Check sheet for the modelled part. Datum: model origin and axes. Units: mm. A direction names the side the tool comes from. Round coordinates to 2 decimals unless told otherwise and drop trailing zeros. Loops run counter-clockwise (first coordinate to the right, second up) from the corner with the lowest first, then second, coordinate; pieces in that order, holes last. Notation, with made-up numbers: (-27.75, -3.5) -> (18.25, -3.5) arc R26 cw to (18.25, 24.5) -> close; hole circle Ø2 at (48, -16.5). An arc over 180 degrees is marked (long way). One line per item, written item: value. Start each with the question number.
1. Release check for a two-part mould opening along X. For faces 1 (the face through (2.01, 3.46, 0.99)), 2 (the face through (-4.8, 1.67, 0.99)), 3 (the face through (-1.99, 3.47, 0.99)), 4 (the face through (0, 6, 1)) record: +X half, -X half, draft (parallel to the pull), parting line (faces both ways), or undercut.
2. Cross-section at D-D on y = -3. Record the cut outline in (x, z), then the cut area to 3 significant figures.
3. Set-up check for faces 5 (the face through (-4.77, -1.64, 0.99)), 6 (the face through (3.84, 3.32, 0.99)), 7 (the face through (4.77, 1.64, 0.99)): record each of +Z, -Z, +X, -X, +Y, -Y from which the full face is reachable in a straight line by a thin tool's end or side.
4. Material ranges on L1, parallel to Y at x = 0, z = 0.8; L2, parallel to Y at x = -4.5, z = 1.9; L3, parallel to X at y = 5, z = 1.85, recorded low to high.
5. Cross-section at B-B on z = 1.4. Record the cut outline in (x, y).
6. Cross-section at A-A on x = 0. Record the cut outline in (y, z), then the cut area to 3 significant figures.
7. Cross-section at C-C on y = 0.5. Record the cut outline in (x, z).
8. Go/stop test with a flat-tipped pin: pin 1 (1.8 mm diameter, centred on x = 0, y = 0, fed in from -Z). Record where the tip stops, or that it passes through.
from build123d import *

# Parameters (mm, degrees)
F1_DEPTH = 2
F2_R     = 1
F3_DEPTH = 2.001


with BuildPart() as f1:
    # F0 (on Top) → F1 (new body)
    with BuildSketch(Plane.XY):
        with BuildLine():
            ThreePointArc((3.877013, -0.984261), (3.969134, -0.495958), (4, 0))
            ThreePointArc((4, 0), (3.969134, 0.495958), (3.877013, 0.984261))
            ThreePointArc((3.877013, 0.984261), (3.464102, 2), (2.790902, 2.865461))
            ThreePointArc((2.790902, 2.865461), (2, 3.464102), (1.086111, 3.849722))
            ThreePointArc((1.086111, 3.849722), (0.548229, 3.962252), (0, 4))
            ThreePointArc((0, 4), (-0.548229, 3.962252), (-1.086111, 3.849722))
            ThreePointArc((-1.086111, 3.849722), (-2, 3.464102), (-2.790902, 2.865461))
            ThreePointArc((-2.790902, 2.865461), (-3.464102, 2), (-3.877013, 0.984261))
            ThreePointArc((-3.877013, 0.984261), (-4, 0), (-3.877013, -0.984261))
            ThreePointArc((-3.877013, -0.984261), (-3.464102, -2), (-2.790902, -2.865461))
            ThreePointArc((-2.790902, -2.865461), (-2, -3.464102), (-1.086111, -3.849722))
            ThreePointArc((-1.086111, -3.849722), (0, -4), (1.086111, -3.849722))
            ThreePointArc((1.086111, -3.849722), (2, -3.464102), (2.790902, -2.865461))
            ThreePointArc((2.790902, -2.865461), (3.464102, -2), (3.877013, -0.984261))
        make_face()
        with BuildLine():
            ThreePointArc((2.790902, 2.865461), (3.464102, 2), (3.877013, 0.984261))
            ThreePointArc((3.877013, 0.984261), (4.783962, 1.654296), (5.446152, 2.566987))
            Line((5.446152, 2.566987), (5.196152, 3))
            Line((5.196152, 3), (4.946152, 3.433013))
            ThreePointArc((4.946152, 3.433013), (3.824643, 3.315885), (2.790902, 2.865461))
        make_face()
        with BuildLine():
            ThreePointArc((5.446152, -2.566987), (4.783962, -1.654296), (3.877013, -0.984261))
            ThreePointArc((3.877013, -0.984261), (3.464102, -2), (2.790902, -2.865461))
            ThreePointArc((2.790902, -2.865461), (3.824643, -3.315885), (4.946152, -3.433013))
            Line((4.946152, -3.433013), (5.196152, -3))
            Line((5.196152, -3), (5.446152, -2.566987))
        make_face()
        with BuildLine():
            ThreePointArc((0, 4), (0.548229, 3.962252), (1.086111, 3.849722))
            ThreePointArc((1.086111, 3.849722), (0.959319, 4.97018), (0.5, 6))
            Line((0.5, 6), (0, 6))
            Line((0, 6), (0, 4))
        make_face()
        with BuildLine():
            ThreePointArc((0.5, -6), (0.959319, -4.97018), (1.086111, -3.849722))
            ThreePointArc((1.086111, -3.849722), (0, -4), (-1.086111, -3.849722))
            ThreePointArc((-1.086111, -3.849722), (-0.959319, -4.97018), (-0.5, -6))
            Line((-0.5, -6), (0, -6))
            Line((0, -6), (0.5, -6))
        make_face()
        with BuildLine():
            ThreePointArc((-1.086111, 3.849722), (-0.548229, 3.962252), (0, 4))
            Line((0, 4), (0, 6))
            Line((0, 6), (-0.5, 6))
            ThreePointArc((-0.5, 6), (-0.959319, 4.97018), (-1.086111, 3.849722))
        make_face()
        with BuildLine():
            ThreePointArc((-4.946152, -3.433013), (-3.824643, -3.315885), (-2.790902, -2.865461))
            ThreePointArc((-2.790902, -2.865461), (-3.464102, -2), (-3.877013, -0.984261))
            ThreePointArc((-3.877013, -0.984261), (-4.783962, -1.654296), (-5.446152, -2.566987))
            Line((-5.446152, -2.566987), (-5.196152, -3))
            Line((-5.196152, -3), (-4.946152, -3.433013))
        make_face()
        with BuildLine():
            ThreePointArc((-3.877013, 0.984261), (-3.464102, 2), (-2.790902, 2.865461))
            ThreePointArc((-2.790902, 2.865461), (-3.824643, 3.315885), (-4.946152, 3.433013))
            Line((-4.946152, 3.433013), (-5.196152, 3))
            Line((-5.196152, 3), (-5.446152, 2.566987))
            ThreePointArc((-5.446152, 2.566987), (-4.783962, 1.654296), (-3.877013, 0.984261))
        make_face()
    extrude(amount=F1_DEPTH)

    # F2 (on face) → F3 (cut, through all)
    with BuildSketch(Plane.XY.offset(2)):
        Circle(F2_R)
    extrude(amount=-F3_DEPTH, mode=Mode.SUBTRACT)


solid = f1.part
Taken from the geometry:
1. face 1: undercut
1. face 2: -X half
1. face 3: undercut
1. face 4: draft
2. outline: (-5.2, 0) -> (-3.02, 0) -> (-3.02, 2) -> (-5.2, 2) -> close; (-2.65, 0) -> (2.65, 0) -> (2.65, 2) -> (-2.65, 2) -> close; (3.02, 0) -> (5.2, 0) -> (5.2, 2) -> (3.02, 2) -> close
2. area: 19.3 mm2
3. face 5: +Z, -Z, -X
3. face 6: +Z, -Z, +Y
3. face 7: +Z, -Z, +X
4. L1: y = -6 to -1, 1 to 6
4. L2: y = -3.43 to -1.4, 1.4 to 3.43
4. L3: x = -0.95 to 0.95
5. outline: (-5.45, -2.57) -> (-4.95, -3.43) arc R3.69 ccw to (-2.79, -2.87) arc R4 ccw to (-1.09, -3.85) arc R3.69 ccw to (-0.5, -6) -> (0.5, -6) arc R3.69 ccw to (1.09, -3.85) arc R4 ccw to (2.79, -2.87) arc R3.69 ccw to (4.95, -3.43) -> (5.45, -2.57) arc R3.69 ccw to (3.88, -0.98) arc R4 ccw to (4, 0) arc R4 ccw to (3.88, 0.98) arc R3.69 ccw to (5.45, 2.57) -> (4.95, 3.43) arc R3.69 ccw to (2.79, 2.87) arc R4 ccw to (1.09, 3.85) arc R3.69 ccw to (0.5, 6) -> (-0.5, 6) arc R3.69 ccw to (-1.09, 3.85) arc R4 ccw to (-2.79, 2.87) arc R3.69 ccw to (-4.95, 3.43) -> (-5.45, 2.57) arc R3.69 ccw to (-3.88, 0.98) arc R4 ccw to (-3.88, -0.98) arc R3.69 ccw to start; hole circle Ø2 at (0, 0)
6. outline: (-6, 0) -> (-1, 0) -> (-1, 2) -> (-6, 2) -> close; (1, 0) -> (6, 0) -> (6, 2) -> (1, 2) -> close
6. area: 20.0 mm2
7. outline: (-3.97, 0) -> (-0.87, 0) -> (-0.87, 2) -> (-3.97, 2) -> close; (0.87, 0) -> (3.97, 0) -> (3.97, 2) -> (0.87, 2) -> close
8. pin 1: passes through
